```python
from build123d import *

# Parameters (mm, degrees)
SKETCH1_W           = 20.2
SKETCH1_H           = 6.4135
BOSS_EXTRUDE1_DEPTH = 6.35
CUT_EXTRUDE1_DEPTH  = 7.35


with BuildPart() as part:
    # Sketch1 → Boss-Extrude1 (new body)
    with BuildSketch(Plane(origin=(0, 0, 0), x_dir=(1, 0, 0), z_dir=(0, 1, 0))):
        with BuildLine():
            ThreePointArc((48.846590956, 16.4135), (0, 51.5305), (-48.846590956, 16.4135))
            Line((-48.846590956, 16.4135), (-39.8, 16.4135))
            Line((-39.8, 16.4135), (-39.8, 10))
            Line((-39.8, 10), (-50.55088951, 10))
            ThreePointArc((-50.55088951, 10), (-51.5305, 0), (-50.55088951, -10))
            Line((-50.55088951, -10), (-39.8, -10))
            Line((-39.8, -10), (-39.8, -16.4135))
            Line((-39.8, -16.4135), (-48.846590956, -16.4135))
            ThreePointArc((-48.846590956, -16.4135), (0, -51.5305), (48.846590956, -16.4135))
            Line((48.846590956, -16.4135), (40, -16.4135))
            Line((40, -16.4135), (40, -10))
            Line((40, -10), (50.55088951, -10))
            ThreePointArc((50.55088951, -10), (51.285012636, -5.023933636), (51.5305, 0))
            ThreePointArc((51.5305, 0), (51.285012636, 5.023933636), (50.55088951, 10))
            Line((50.55088951, 10), (40, 10))
            Line((40, 10), (40, 16.4135))
            Line((40, 16.4135), (48.846590956, 16.4135))
        make_face()
        with Locations((0.1, -13.20675)):
            Rectangle(SKETCH1_W, SKETCH1_H, mode=Mode.SUBTRACT)
        with Locations((0.1, 13.20675)):
            Rectangle(SKETCH1_W, SKETCH1_H, mode=Mode.SUBTRACT)
    extrude(amount=BOSS_EXTRUDE1_DEPTH)

    # Sketch2 → Cut-Extrude1 (cut, through all)
    with BuildSketch(Plane(origin=(0, 6.35, 0), x_dir=(1, 0, 0), z_dir=(0, 1, 0))):
        with BuildLine():
            ThreePointArc((-27.13748547, -27.13748547), (0, -38.3782), (27.13748547, -27.13748547))
            ThreePointArc((27.13748547, -27.13748547), (27.13748547, -22.359989213), (22.359989213, -22.359989213))
            ThreePointArc((22.359989213, -22.359989213), (0, -31.6218), (-22.359989213, -22.359989213))
            ThreePointArc((-22.359989213, -22.359989213), (-27.13748547, -22.359989213), (-27.13748547, -27.13748547))
        make_face()
        with BuildLine():
            ThreePointArc((-27.13748547, 27.13748547), (0, 38.3782), (27.13748547, 27.13748547))
            ThreePointArc((27.13748547, 27.13748547), (27.13748547, 22.359989213), (22.359989213, 22.359989213))
            ThreePointArc((22.359989213, 22.359989213), (0, 31.6218), (-22.359989213, 22.359989213))
            ThreePointArc((-22.359989213, 22.359989213), (-27.13748547, 22.359989213), (-27.13748547, 27.13748547))
        make_face()
    extrude(amount=-CUT_EXTRUDE1_DEPTH, mode=Mode.SUBTRACT)


solid = part.part
```
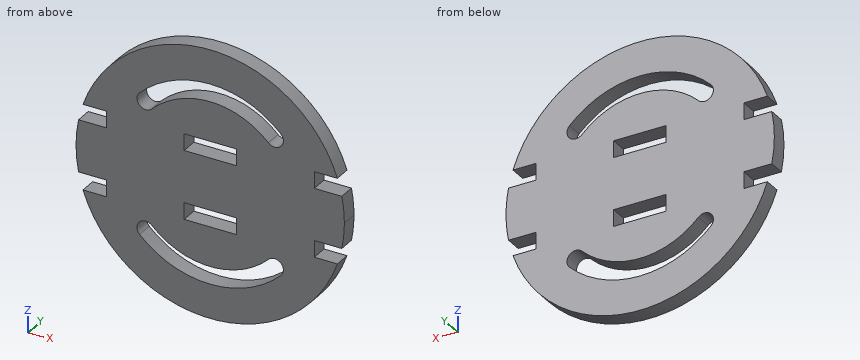
For this review, take the finished solid that the model builds, in its own axes (mm). Round coordinates to 2 decimals unless told otherwise and drop trailing zeros. Write each loop counter-clockwise with the first axis right and the second up, starting at its lowest first coordinate (ties: lowest second). Pieces come first, ordered by that corner, then holes. Notation, with made-up numbers: (23.5, -24.75) -> (76.5, -24.75) arc R14 cw to (76.5, 1.25) -> close; hole circle Ø10 at (-27.5, -24). An arc over 180 degrees is marked (long way). One line per question, with ' | ' between items. Start each with the question number.
1) Add section A-A (z = 34.5). Write out the cut boundary in (x, y), and give its area (3 significant figures).
2) Add section C-C (x = -8). Write out the cut boundary in (y, z).
3) Wall thickness on line 1 along X through (y, z) = (3, -11); line 2 along Z through (x, y) = (-46, 1); line 3 along Z through (x, y) = (-22.5, 1.75): over which ranges is each line inside the solid? List them lowest first.
4) Add section B-B (y = 2). Count the separate pieces of the cut face and the enclosed holes in it, and give its area (3 significant figures).
5) For pin 1 Ø3 at (x, y) = (43.5, 2) entering from -Z; pin 2 Ø12 at (x, z) = (-23, 15) entering from -Y; pin 3 Ø1.9 at (x, y) = (45.5, 4.5) entering from -Z; pin 4 Ø1.9 at (y, z) = (4, -12) entering from +X, all flat-tipped, find the tip position at first contact; note any pin that passes through.
6) Add section D-D (x = -45). Write out the cut boundary in (y, z), and give its area (3 significant figures).
Reported:
1) outline: (-38.28, 0) -> (-16.81, 0) -> (-16.81, 6.35) -> (-38.28, 6.35) -> close; (16.81, 0) -> (38.28, 0) -> (38.28, 6.35) -> (16.81, 6.35) -> close | area: 273 mm²
2) outline: (0, -50.91) -> (6.35, -50.91) -> (6.35, -37.54) -> (0, -37.54) -> close; (0, -30.59) -> (6.35, -30.59) -> (6.35, -16.41) -> (0, -16.41) -> close; (0, -10) -> (6.35, -10) -> (6.35, 10) -> (0, 10) -> close; (0, 16.41) -> (6.35, 16.41) -> (6.35, 30.59) -> (0, 30.59) -> close; (0, 37.54) -> (6.35, 37.54) -> (6.35, 50.91) -> (0, 50.91) -> close
3) line 1: x = -39.8 to -10, 10.2 to 40 | line 2: z = -23.22 to -16.41, -10 to 10, 16.41 to 23.22 | line 3: z = -46.36 to -31.09, -22.23 to 22.23, 31.09 to 46.36
4) separate pieces: 1 | enclosed holes: 4 | area: 7,020 mm²
5) pin 1: stops at z = -29.86 | pin 2: stops at y = 0 | pin 3: stops at z = -25.9 | pin 4: stops at x = 40
6) outline: (0, -25.11) -> (6.35, -25.11) -> (6.35, -16.41) -> (0, -16.41) -> close; (0, -10) -> (6.35, -10) -> (6.35, 10) -> (0, 10) -> close; (0, 16.41) -> (6.35, 16.41) -> (6.35, 25.11) -> (0, 25.11) -> close | area: 237 mm²
